The listing builds one solid part. Answer for the finished solid, in the listing's coordinates (mm). A direction names the side the tool comes from. Coordinates: 2 decimals unless noted, no trailing zeros. Loops run counter-clockwise (first coordinate to the right, second up) from the corner with the lowest first, then second, coordinate; pieces in that order, holes last. Notation, with made-up numbers: M 4,57 L 46,57 A18 cw 46,72 Z; hole C 35,23.25 d7. An arc over 180 degrees is marked long. Answer as a JSON object with one key per item and string values. Group by question number.
1. Determine the mould class of faces 1 (the face through (47.15, 5.07, 126.99)), 2 (the face through (-1, 10, 34)), 3 (the face through (0.66, 4.93, -14.985)) for opening direction Z: released by +Z, released by -Z, zero draft, split by the parting line, or undercut.
2. Straight lines are drawn through the part: L1, parallel to Z at x = -40, y = 6.5; L2, parallel to X at y = 7, z = 120; L3, parallel to X at y = 6.25, z = 10. For each, find the intervals that lie inside material, in ascending order.
3. A cutting plane is placed at B-B on z = 0. Give the vertices of the cut face in (x, y), and give its area (3 significant figures).
4. For faces 4 (the face through (-1, 0, 34)), 5 (the face through (26.99, 5.07, 82.85)), determine the directions among +Z, -Z, +X, -X, +Y, -Y from which every point of the face is accessible in a straight line to the end or side of a thin tool.
5. A cutting plane is placed at C-C on y = 6.5. State how many separate pieces and enclosed holes the cut face has, and give its area (3 significant figures).
6. A cutting plane is placed at A-A on x = 0. Give the vertices of the cut face in (y, z).
7. Given pin 1 (1.9 mm diameter, centred on x = 40, z = 90, fed in from -Y), flat-ended and moving along its own axis, determine where the tip first touches the part or whether it passes through.
from build123d import *

# Parameters (mm, degrees)
BOSS_EXTRUDE1_DEPTH     = 10
CUT_EXTRUDE1_DEPTH      = 140.642400438
CUT_EXTRUDE1_DEPTH_BACK = 140.642400438
SKETCH2_R               = 15
SKETCH2_R_2             = 1.6
CUT_EXTRUDE2_DEPTH      = 140.642400438
CUT_EXTRUDE2_DEPTH_BACK = 140.642400438
SKETCH3_W               = 60
SKETCH3_H               = 50
CUT_EXTRUDE3_DEPTH      = 140.642400438
CUT_EXTRUDE3_DEPTH_BACK = 140.642400438
SKETCH4_R               = 1.6
FILLET1_R               = 10


with BuildPart() as part:
    # Sketch1 → Boss-Extrude1 (new body)
    with BuildSketch(Plane(origin=(0, 0, 0), x_dir=(1, 0, 0), z_dir=(0, 1, 0))):
        Polygon((-50, -60), (-50, -130), (50, -130), (50, -60), (50, 60), (-50, 60), align=None)
    extrude(amount=BOSS_EXTRUDE1_DEPTH)

    # Sketch2 → Cut-Extrude1 (cut, two sides: drawn at the far end of the back side and taken through both)
    with BuildSketch(Plane(origin=(0, 10, 0), x_dir=(1, 0, 0), z_dir=(0, 1, 0)).offset(-CUT_EXTRUDE1_DEPTH_BACK)):
        with Locations(Location((0, 0, 0), (0, 0, 270))):
            Circle(SKETCH2_R)
        with Locations(Location((-40, -50, 0), (0, 0, 270))):
            Circle(SKETCH2_R_2)
        with Locations(Location((40, -50, 0), (0, 0, 270))):
            Circle(SKETCH2_R_2)
        with Locations(Location((40, 50, 0), (0, 0, 270))):
            Circle(SKETCH2_R_2)
        with Locations(Location((-40, 50, 0), (0, 0, 270))):
            Circle(SKETCH2_R_2)
        with Locations(Location((-40, -120, 0), (0, 0, 270))):
            Circle(SKETCH2_R_2)
        with Locations(Location((40, -120, 0), (0, 0, 270))):
            Circle(SKETCH2_R_2)
        with Locations(Location((-40, -90, 0), (0, 0, 270))):
            Circle(SKETCH2_R_2)
        with Locations(Location((40, -90, 0), (0, 0, 270))):
            Circle(SKETCH2_R_2)
    extrude(amount=CUT_EXTRUDE1_DEPTH + CUT_EXTRUDE1_DEPTH_BACK, mode=Mode.SUBTRACT)

    # Sketch3 → Cut-Extrude2 (cut, two sides: drawn at the far end of the back side and taken through both)
    with BuildSketch(Plane(origin=(0, 10, 0), x_dir=(1, 0, 0), z_dir=(0, 1, 0)).offset(-CUT_EXTRUDE2_DEPTH_BACK)):
        with Locations((0, -105)):
            Rectangle(SKETCH3_W, SKETCH3_H)
    extrude(amount=CUT_EXTRUDE2_DEPTH + CUT_EXTRUDE2_DEPTH_BACK, mode=Mode.SUBTRACT)

    # Sketch4 → Cut-Extrude3 (cut, two sides: drawn at the far end of the back side and taken through both)
    with BuildSketch(Plane(origin=(0, 10, 0), x_dir=(1, 0, 0), z_dir=(0, 1, 0)).offset(-CUT_EXTRUDE3_DEPTH_BACK)):
        with Locations(Location((-30, 10, 0), (0, 0, 270))):
            Circle(SKETCH4_R)
        with Locations(Location((-30, -10, 0), (0, 0, 270))):
            Circle(SKETCH4_R)
        with Locations(Location((30, 10, 0), (0, 0, 270))):
            Circle(SKETCH4_R)
        with Locations(Location((30, -10, 0), (0, 0, 270))):
            Circle(SKETCH4_R)
    extrude(amount=CUT_EXTRUDE3_DEPTH + CUT_EXTRUDE3_DEPTH_BACK, mode=Mode.SUBTRACT)

    # Fillet1
    fillet1_edges = [part.edges().sort_by_distance(p)[0] for p in [
        (50, 5, -60),
        (-50, 5, -60),
        (-50, 5, 130),
        (-30, 5, 130),
        (50, 5, 130),
        (30, 5, 130),
        (30, 5, 80),
        (-30, 5, 80),
    ]]
    fillet(fillet1_edges, radius=FILLET1_R - 0.0001)  # a hair under: the kernel refuses the full size


solid = part.part
From the geometry:
{
 "1": {"face 1": "released by +Z", "face 2": "zero draft", "face 3": "undercut"},
 "2": {"L1": "z = -60 to -51.6, -48.4 to 48.4, 51.6 to 88.4, 91.6 to 118.4, 121.6 to 130", "L2": "x = -50 to -41.6, -38.4 to -30, 30 to 38.4, 41.6 to 50", "L3": "x = -50 to -31.6, -28.4 to -11.18, 11.18 to 28.4, 31.6 to 50"},
 "3": {"outline": "M -50,0 L -15,0 L -15,10 L -50,10 Z; M 15,0 L 50,0 L 50,10 L 15,10 Z", "area": "700 mm²"},
 "4": {"face 4": "+Z, -Z, +X, -X, -Y", "face 5": "+Z, +Y, -Y"},
 "5": {"separate pieces": "1", "enclosed holes": "13", "area": "15,100 mm²"},
 "6": {"outline": "M 0,-60 L 10,-60 L 10,-15 L 0,-15 Z; M 0,15 L 10,15 L 10,80 L 0,80 Z"},
 "7": {"pin 1": "passes through"}
}
